```python
from build123d import *

# Parameters (mm, degrees)
BOSS_EXTRUDE1_DEPTH       = 7.3
SKETCH2_R                 = 2.475
CUT_EXTRUDE1_DEPTH        = 53.555779891
SKETCH3_R                 = 3.125
CUT_EXTRUDE2_DEPTH        = 0.85
LPATTERN1_COUNT           = 7
LPATTERN1_PITCH           = 8
LPATTERN1_COPY_1_SKETCH_R = 3.125
LPATTERN1_COPY_1_DEPTH    = 0.85
LPATTERN1_COPY_2_SKETCH_R = 3.125
LPATTERN1_COPY_2_DEPTH    = 0.85
LPATTERN1_COPY_3_SKETCH_R = 3.125
LPATTERN1_COPY_3_DEPTH    = 0.85
LPATTERN1_COPY_4_SKETCH_R = 3.125
LPATTERN1_COPY_4_DEPTH    = 0.85
LPATTERN1_COPY_5_SKETCH_R = 3.125
LPATTERN1_COPY_5_DEPTH    = 0.85
LPATTERN1_COPY_6_SKETCH_R = 3.125
LPATTERN1_COPY_6_DEPTH    = 0.85
CHAMFER1_SIZE             = 0.4


with BuildPart() as part:
    # Sketch1 → Boss-Extrude1 (new body)
    with BuildSketch(Plane(origin=(0, 0, 0), x_dir=(1, 0, 0), z_dir=(0, 1, 0))):
        with BuildLine():
            Line((0, 3.9), (48, 3.9))
            ThreePointArc((48, 3.9), (51.9, 0), (48, -3.9))
            Line((48, -3.9), (0, -3.9))
            ThreePointArc((0, -3.9), (-3.9, 0), (0, 3.9))
        make_face()
    extrude(amount=BOSS_EXTRUDE1_DEPTH)

    # Sketch2 → Cut-Extrude1 (cut, through all)
    with BuildSketch(Plane(origin=(0, 7.3, 0), x_dir=(1, 0, 0), z_dir=(0, 1, 0))):
        with Locations(Location((0, 0, 0), (0, 0, 270))):
            Circle(SKETCH2_R)
    cut_extrude1 = extrude(amount=-CUT_EXTRUDE1_DEPTH, mode=Mode.SUBTRACT)

    # Sketch3 → Cut-Extrude2 (cut)
    with BuildSketch(Plane(origin=(0, 7.3, 0), x_dir=(1, 0, 0), z_dir=(0, 1, 0))):
        with Locations(Location((0, 0, 0), (0, 0, 270))):
            Circle(SKETCH3_R)
    cut_extrude2 = extrude(amount=-CUT_EXTRUDE2_DEPTH, mode=Mode.SUBTRACT)

    # Mirror1: Cut-Extrude2 across plane
    add(cut_extrude2.mirror(Plane.ZX.offset(3.65)), mode=Mode.SUBTRACT)

    # LPattern1: Cut-Extrude1, Cut-Extrude2 ×7
    with Locations(*[(i * LPATTERN1_PITCH, 0, 0) for i in range(1, LPATTERN1_COUNT)]):
        add(cut_extrude1, mode=Mode.SUBTRACT)
        add(cut_extrude2, mode=Mode.SUBTRACT)

    # LPattern1 copy 1 sketch → LPattern1 copy 1 (cut)
    with BuildSketch(Plane(origin=(8, 0, 0), x_dir=(1, 0, 0), z_dir=(0, -1, 0))):
        Circle(LPATTERN1_COPY_1_SKETCH_R)
    extrude(amount=-LPATTERN1_COPY_1_DEPTH, mode=Mode.SUBTRACT)

    # LPattern1 copy 2 sketch → LPattern1 copy 2 (cut)
    with BuildSketch(Plane(origin=(16, 0, 0), x_dir=(1, 0, 0), z_dir=(0, -1, 0))):
        Circle(LPATTERN1_COPY_2_SKETCH_R)
    extrude(amount=-LPATTERN1_COPY_2_DEPTH, mode=Mode.SUBTRACT)

    # LPattern1 copy 3 sketch → LPattern1 copy 3 (cut)
    with BuildSketch(Plane(origin=(24, 0, 0), x_dir=(1, 0, 0), z_dir=(0, -1, 0))):
        Circle(LPATTERN1_COPY_3_SKETCH_R)
    extrude(amount=-LPATTERN1_COPY_3_DEPTH, mode=Mode.SUBTRACT)

    # LPattern1 copy 4 sketch → LPattern1 copy 4 (cut)
    with BuildSketch(Plane(origin=(32, 0, 0), x_dir=(1, 0, 0), z_dir=(0, -1, 0))):
        Circle(LPATTERN1_COPY_4_SKETCH_R)
    extrude(amount=-LPATTERN1_COPY_4_DEPTH, mode=Mode.SUBTRACT)

    # LPattern1 copy 5 sketch → LPattern1 copy 5 (cut)
    with BuildSketch(Plane(origin=(40, 0, 0), x_dir=(1, 0, 0), z_dir=(0, -1, 0))):
        Circle(LPATTERN1_COPY_5_SKETCH_R)
    extrude(amount=-LPATTERN1_COPY_5_DEPTH, mode=Mode.SUBTRACT)

    # LPattern1 copy 6 sketch → LPattern1 copy 6 (cut)
    with BuildSketch(Plane(origin=(48, 0, 0), x_dir=(1, 0, 0), z_dir=(0, -1, 0))):
        Circle(LPATTERN1_COPY_6_SKETCH_R)
    extrude(amount=-LPATTERN1_COPY_6_DEPTH, mode=Mode.SUBTRACT)

    # Chamfer1
    # the kernel refuses this chamfer: 0.4 mm, written as the material it takes off along each edge
    with BuildSketch(Plane(origin=(16, 0, 0), x_dir=(1, 0, 0), z_dir=(0, 0, -1))) as chamfer1_piece_1:
        Polygon((3.125 + CHAMFER1_SIZE, 0), (3.125, -CHAMFER1_SIZE), (3.125, 0), align=None)
    revolve(axis=Axis((16, 0, 0), (0, -1, 0)), mode=Mode.SUBTRACT)
    with BuildSketch(Plane(origin=(24, 0, 0), x_dir=(1, 0, 0), z_dir=(0, 0, -1))) as chamfer1_piece_2:
        Polygon((3.125 + CHAMFER1_SIZE, 0), (3.125, -CHAMFER1_SIZE), (3.125, 0), align=None)
    revolve(axis=Axis((24, 0, 0), (0, -1, 0)), mode=Mode.SUBTRACT)
    with BuildSketch(Plane(origin=(32, 0, 0), x_dir=(1, 0, 0), z_dir=(0, 0, -1))) as chamfer1_piece_3:
        Polygon((3.125 + CHAMFER1_SIZE, 0), (3.125, -CHAMFER1_SIZE), (3.125, 0), align=None)
    revolve(axis=Axis((32, 0, 0), (0, -1, 0)), mode=Mode.SUBTRACT)
    with BuildSketch(Plane(origin=(40, 0, 0), x_dir=(1, 0, 0), z_dir=(0, 0, -1))) as chamfer1_piece_4:
        Polygon((3.125 + CHAMFER1_SIZE, 0), (3.125, -CHAMFER1_SIZE), (3.125, 0), align=None)
    revolve(axis=Axis((40, 0, 0), (0, -1, 0)), mode=Mode.SUBTRACT)
    with BuildSketch(Plane(origin=(48, 0, 0), x_dir=(1, 0, 0), z_dir=(0, 0, -1))) as chamfer1_piece_5:
        Polygon((3.125 + CHAMFER1_SIZE, 0), (3.125, -CHAMFER1_SIZE), (3.125, 0), align=None)
    revolve(axis=Axis((48, 0, 0), (0, -1, 0)), mode=Mode.SUBTRACT)
    with BuildSketch(Plane(origin=(0, 0, 0), x_dir=(0, 0, 1), z_dir=(-1, 0, 0))) as chamfer1_piece_6:
        Polygon((3.125 + CHAMFER1_SIZE, 0), (3.125, CHAMFER1_SIZE), (3.125, 0), align=None)
    revolve(axis=Axis((0, 0, 0), (0, 1, 0)), mode=Mode.SUBTRACT)
    with BuildSketch(Plane(origin=(0, 0, -3.9), x_dir=(0, 0.9996219169112968, -0.027495876610586275), z_dir=(1, 0, 0))) as chamfer1_piece_7:
        Polygon((CHAMFER1_SIZE * 0.999621916911, CHAMFER1_SIZE * 0.0274958766106), (-CHAMFER1_SIZE * 0.0274958766106, CHAMFER1_SIZE * 0.999621916911), (0, 0), align=None)
    extrude(amount=48, mode=Mode.SUBTRACT)
    with BuildSketch(Plane(origin=(48, 0, 0), x_dir=(0, 0, -1), z_dir=(-1, 0, 0))) as chamfer1_piece_8:
        Polygon((3.9, -CHAMFER1_SIZE), (3.9 - CHAMFER1_SIZE, 0), (3.9, 0), align=None)
    revolve(axis=Axis((48, 0, 0), (0, -1, 0)), revolution_arc=180, mode=Mode.SUBTRACT)
    with BuildSketch(Plane(origin=(48, 0, 3.9), x_dir=(0, -0.027495876610586386, -0.9996219169112968), z_dir=(-1, 0, 0))) as chamfer1_piece_9:
        Polygon((CHAMFER1_SIZE * 0.999621916911, -CHAMFER1_SIZE * 0.0274958766106), (-CHAMFER1_SIZE * 0.0274958766106, -CHAMFER1_SIZE * 0.999621916911), (0, 0), align=None)
    extrude(amount=48, mode=Mode.SUBTRACT)
    with BuildSketch(Plane(origin=(0, 0, 0), x_dir=(0, 0, 1), z_dir=(1, 0, 0))) as chamfer1_piece_10:
        Polygon((3.9, -CHAMFER1_SIZE), (3.9 - CHAMFER1_SIZE, 0), (3.9, 0), align=None)
    revolve(axis=Axis((0, 0, 0), (0, -1, 0)), revolution_arc=180, mode=Mode.SUBTRACT)
    with BuildSketch(Plane(origin=(8, 0, 0), x_dir=(1, 0, 0), z_dir=(0, 0, -1))) as chamfer1_piece_11:
        Polygon((3.125 + CHAMFER1_SIZE, 0), (3.125, -CHAMFER1_SIZE), (3.125, 0), align=None)
    revolve(axis=Axis((8, 0, 0), (0, -1, 0)), mode=Mode.SUBTRACT)


solid = part.part
```
Model file for the job. Use its own axes, mm. A direction names the side the tool comes from. Give positions to 0.01 mm unless a question says otherwise; leave off trailing zeros. Order: outer loops, then holes, each group sorted by start corner. A loop starts at its lowest first (then second) coordinate and runs counter-clockwise, first axis right, second up.
1) Wall check: probe 1 along Z at (x, y) = (16, 0.6) (3 decimals); probe 2 along Z at (x, y) = (9, 3.25); probe 3 along Y at (x, z) = (29.5, -1.25). Give the ranges that are in metal, low to high.
2) 3-axis set-ups, long thin cutter, end or side, ignore diameter. For faces 1 (the flat face through (12, 0, 0)), 2 (the cylindrical face through (35.1, 6.9, -0.4)), 3 (the cylindrical face through (50.98, 0.62, 0.94)): which of +Z, -Z, +X, -X, +Y, -Y reach the whole face in a straight line?
3) Saw through at B-B, the plane z = -0.5. Count the separate pieces of the cut face and the enclosed holes in it, then the cut area to 3 significant figures.
4) Saw through at A-A, the plane y = 4.25. Write the cut outline in (x, z) (3 decimals).
5) Pin check, flat tips, straight feed: pin 1 (3 mm diameter, centred on x = 9, z = -0.5, fed in from -Y); pin 2 (4 mm diameter, centred on x = 10.5, z = -0.5, fed in from +Y). Stop position of each tip, or through.
6) Mould opens along X. For faces 4 (the cylindrical face through (19.1, 6.9, -0.4)), 5 (the cylindrical face through (51.9, 3.8, -0.1)), 6 (the flat face through (36, 0, 0)) say: +X half, -X half, draft (parallel to the pull), parting line (faces both ways), or undercut.
Computed:
1. probe 1: z = -3.9 to -3.125, 3.125 to 3.9
1. probe 2: z = -3.9 to -2.26, 2.26 to 3.9
1. probe 3: y = 0.85 to 6.45
2. face 1: +Z, -Z, +X, -X, -Y
2. face 2: +Y
2. face 3: -Y
3. separate pieces: 8
3. enclosed holes: 0
3. area: 142 mm2
4. outline: (0, -3.9) - (48, -3.9) arc R3.9 ccw to (48, 3.9) - (0, 3.9) arc R3.9 ccw to start; hole circle Ø4.95 at (0, 0); hole circle Ø4.95 at (8, 0); hole circle Ø4.95 at (16, 0); hole circle Ø4.95 at (24, 0); hole circle Ø4.95 at (32, 0); hole circle Ø4.95 at (40, 0); hole circle Ø4.95 at (48, 0)
5. pin 1: stops at y = 0.85
5. pin 2: stops at y = 7.3
6. face 4: undercut
6. face 5: +X half
6. face 6: draft
